The model under review builds one solid part; all positions refer to its coordinate system, in mm. Face numbers are marked on the shaded views. A direction names the side the tool comes from. Coordinates: 2 decimals unless noted, no trailing zeros. Loops run counter-clockwise (first coordinate to the right, second up) from the corner with the lowest first, then second, coordinate; pieces in that order, holes last. Notation, with made-up numbers: M 54,83.5 L 69,83.5 A30 ccw 69,119.5 Z; hole C 10,-35 d1. An arc over 180 degrees is marked long. Write item = value, one per line. Start each with the question number.
Q1. Mouldability with a two-part tool opening along Y and no side actions: class the marked faces 1, 2, 3 and 4 as released by +Y, released by -Y, zero draft, split by the parting line, or undercut.
Q2. We need section C-C on z = 20. Give the boundary of the cut face in (x, y).
Q3. Clearance check with flat-ended pins moving along their axes: pin 1 Ø4 at (x, y) = (-12, 22) entering from -Z; pin 2 Ø0.8 at (x, z) = (-14.5, 20) entering from +Y; pin 3 Ø8 at (x, y) = (-6.5, -20.5) entering from +Z. State where each tip first meets the part, or that it passes through.
Q4. We need section A-A on x = -15. Give the boundary of the cut face in (y, z), and give its area (3 significant figures).
Q5. We need section B-B on x = 0. Give the boundary of the cut face in (y, z).
Q6. For the marked faces 5 and 6, list the 3-axis set-ups (+Z, -Z, +X, -X, +Y, -Y) from which the entire face can be reached by the end or side of a thin tool; tool diameter is ignored.
Q7. We need section D-D on y = -21. Give the boundary of the cut face in (x, z), and give its area (3 significant figures).
Q8. Wall thickness on probe 1 along X at (y, z) = (34.25, 20); probe 2 along Y at (x, z) = (-1.5, 23.5); probe 3 along Z at (x, y) = (15, -30): over which ranges is each line inside the solid? List them lowest first.
from build123d import *

# Parameters (mm, degrees)
SKETCH1_W                           = 40
SKETCH1_H                           = 75
BOSS_EXTRUDE1_DEPTH                 = 10
SKETCH2_W                           = 40
SKETCH2_H                           = 10
BOSS_EXTRUDE2_DEPTH                 = 15
SKETCH3_R                           = 1.25
CUT_EXTRUDE1_DEPTH                  = 70
FILLET1_R                           = 3
FILLET2_R                           = 3
SKETCH4_R                           = 5.1
CUT_EXTRUDE2_DEPTH                  = 10
ENL_V_MAT_EXTRU_1_REACH             = 62.26
ENL_V_MAT_EXTRU_1_END_RADIUS        = 5.1
ESQUISSE1_R                         = 2.55
ENL_V_MAT_EXTRU_1_DIRECTION_2_DEPTH = 61.259853966
ESQUISSE2_W                         = 2.5
ESQUISSE2_H                         = 5.92504729
ENL_V_MAT_EXTRU_2_DEPTH             = 50.307707349


with BuildPart() as part:
    # Sketch1 → Boss-Extrude1 (new body)
    with BuildSketch(Plane.XY):
        Rectangle(SKETCH1_W, SKETCH1_H)
    extrude(amount=BOSS_EXTRUDE1_DEPTH)

    # Sketch2 → Boss-Extrude2 (add)
    with BuildSketch(Plane.XY.offset(10)):
        with Locations((0, 32.5)):
            Rectangle(SKETCH2_W, SKETCH2_H)
        with Locations((0, -32.5)):
            Rectangle(SKETCH2_W, SKETCH2_H)
    extrude(amount=BOSS_EXTRUDE2_DEPTH)

    # Sketch3 → Cut-Extrude1 (cut)
    with BuildSketch(Plane(origin=(0, 37.5, 0), x_dir=(1, 0, 0), z_dir=(0, 1, 0))):
        with Locations(Location((-15, -20, 0), (0, 0, 270))):
            Circle(SKETCH3_R)
        with Locations(Location((15, -20, 0), (0, 0, 90))):
            Circle(SKETCH3_R)
    extrude(amount=-CUT_EXTRUDE1_DEPTH, mode=Mode.SUBTRACT)

    # Fillet1
    fillet1_edges = [part.edges().sort_by_distance(p)[0] for p in [
        (-20, 32.5, 25),
        (20, 32.5, 25),
    ]]
    fillet(fillet1_edges, radius=FILLET1_R)

    # Fillet2
    fillet2_edges = [part.edges().sort_by_distance(p)[0] for p in [
        (-20, -32.5, 25),
        (20, -32.5, 25),
    ]]
    fillet(fillet2_edges, radius=FILLET2_R)

    # Sketch4 → Cut-Extrude2 (cut)
    with BuildSketch(Plane(origin=(0, 0, 0), x_dir=(-1, 0, 0), z_dir=(0, 0, -1))):
        with Locations((0, -21)):
            Circle(SKETCH4_R)
    extrude(amount=-CUT_EXTRUDE2_DEPTH, mode=Mode.SUBTRACT)

    # Enlèv. mat.-Extru.1: up to this cylinder (the profile starts outside it)
    enl_v_mat_extru_1_end = Plane(origin=(0, -21, 4.63857), z_dir=(0, 0, -1)) * Cylinder(ENL_V_MAT_EXTRU_1_END_RADIUS, 135.72, mode=Mode.PRIVATE)
    # Esquisse1 → Enlèv. mat.-Extru.1 (cut, up to the surface)
    with BuildSketch(Plane.ZY.offset(20), mode=Mode.PRIVATE) as enl_v_mat_extru_1_sk1:
        with Locations(Location((4.63857049, -21, 0), (0, 0, 180))):
            Circle(ESQUISSE1_R)
    enl_v_mat_extru_1_tool1 = extrude(enl_v_mat_extru_1_sk1.sketch, amount=-ENL_V_MAT_EXTRU_1_REACH, mode=Mode.PRIVATE) - enl_v_mat_extru_1_end
    add(enl_v_mat_extru_1_tool1.solids().sort_by_distance((-20, -21, 4.63857))[0], mode=Mode.SUBTRACT)

    # Esquisse1 → Enlèv. mat.-Extru.1 direction 2 (cut)
    with BuildSketch(Plane.ZY.offset(20)):
        with Locations(Location((4.63857049, -21, 0), (0, 0, 180))):
            Circle(ESQUISSE1_R)
    extrude(amount=ENL_V_MAT_EXTRU_1_DIRECTION_2_DEPTH, mode=Mode.SUBTRACT)

    # Esquisse2 → Enlèv. mat.-Extru.2 (cut, through all)
    with BuildSketch(Plane(origin=(0, 0, 0), x_dir=(-1, 0, 0), z_dir=(0, 0, -1))):
        with Locations((8.108583092, -21)):
            Rectangle(ESQUISSE2_W, ESQUISSE2_H)
    extrude(amount=-ENL_V_MAT_EXTRU_2_DEPTH, mode=Mode.SUBTRACT)


solid = part.part
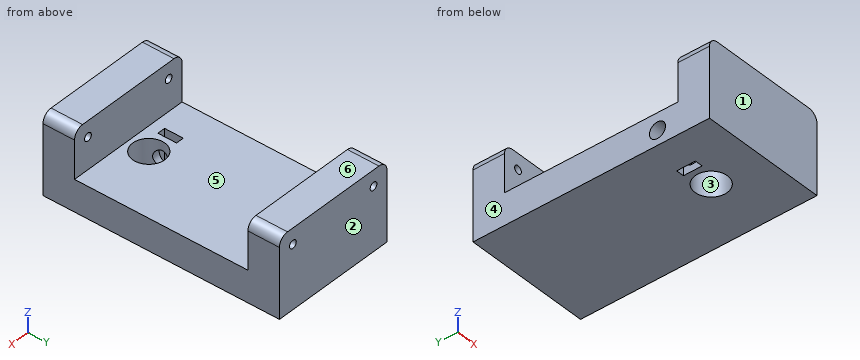
Returned:
q1.face_1 = released by -Y
q1.face_2 = released by +Y
q1.face_3 = undercut
q1.face_4 = zero draft
q2.outline = M -20,-37.5 L 20,-37.5 L 20,-27.5 L 16.25,-27.5 L 16.25,-32.5 L 13.75,-32.5 L 13.75,-27.5 L -13.75,-27.5 L -13.75,-32.5 L -16.25,-32.5 L -16.25,-27.5 L -20,-27.5 Z; M -20,27.5 L -16.25,27.5 L -16.25,37.5 L -20,37.5 Z; M -13.75,27.5 L 13.75,27.5 L 13.75,37.5 L -13.75,37.5 Z; M 16.25,27.5 L 20,27.5 L 20,37.5 L 16.25,37.5 Z
q3.pin_1 = 0
q3.pin_2 = -32.5
q3.pin_3 = 10
q4.outline = M -37.5,0 L 37.5,0 L 37.5,18.75 L 27.5,18.75 L 27.5,10 L -27.5,10 L -27.5,18.75 L -32.5,18.75 L -32.5,21.25 L -27.5,21.25 L -27.5,25 L -37.5,25 Z; M 27.5,21.25 L 37.5,21.25 L 37.5,25 L 27.5,25 Z; hole C -21,4.64 d5.1
q4.area = 992 mm^2
q5.outline = M -37.5,0 L -26.1,0 L -26.1,10 L -27.5,10 L -27.5,25 L -37.5,25 Z; M -15.9,0 L 37.5,0 L 37.5,25 L 27.5,25 L 27.5,10 L -15.9,10 Z
q6.face_5 = +Z, +X, -X
q6.face_6 = +Z, +X, -X, +Y, -Y
q7.outline = M -20,0 L -9.36,0 L -9.36,2.09 L -20,2.09 Z; M -20,7.19 L -9.36,7.19 L -9.36,10 L -20,10 Z; M -6.86,0 L -5.1,0 L -5.1,2.09 L -6.86,2.09 Z; M -6.86,7.19 L -5.1,7.19 L -5.1,10 L -6.86,10 Z; M 5.1,0 L 20,0 L 20,10 L 5.1,10 Z
q7.area = 210 mm^2
q8.probe_1 = -20 to -16.25, -13.75 to 13.75, 16.25 to 20
q8.probe_2 = -37.5 to -27.5, 27.5 to 37.5
q8.probe_3 = 0 to 18.75, 21.25 to 25
